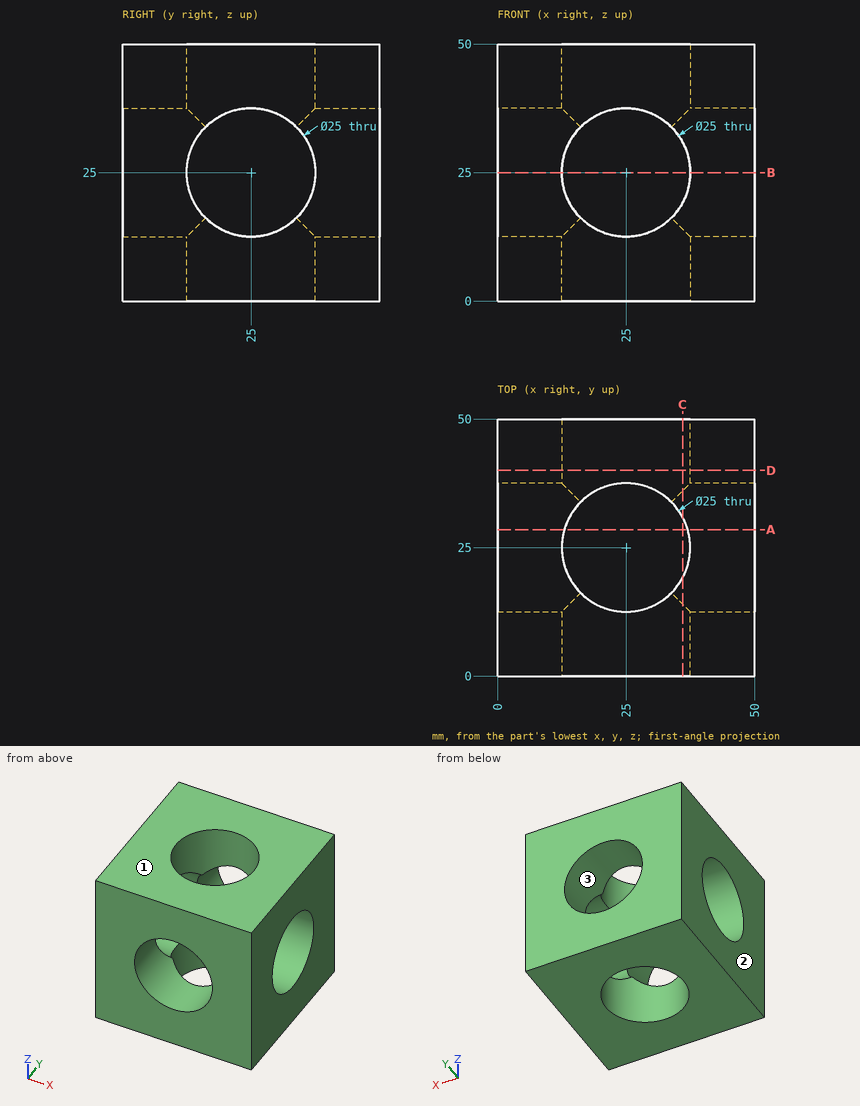
Can you work these out from the drawing? Everything is in mm from the part's minimum corner. Round coordinates to 2 decimals unless told otherwise and drop trailing zeros. Loops run counter-clockwise (first coordinate to the right, second up) from the corner with the lowest first, then second, coordinate; pieces in that order, holes last. Notation, with made-up numbers: (10, 18.25) -> (65, 18.25) arc R7 ccw to (65, 24.25) -> close; hole circle Ø11 at (78, 24). An arc over 180 degrees is marked (long way). Put each result on its own line as item: value.
Q1. I want a section at A-A on y = 28.5. Write out the boundary of the cut face in (x, z), and give its area (3 significant figures).
Checks:
outline: (0, 0) -> (13, 0) -> (13, 13) -> (0, 13) -> close; (0, 37) -> (13, 37) -> (13, 50) -> (0, 50) -> close; (37, 0) -> (50, 0) -> (50, 13) -> (37, 13) -> close; (37, 37) -> (50, 37) -> (50, 50) -> (37, 50) -> close
area: 676 mm2
Q2. I want a section at B-B on z = 25. Write out the boundary of the cut face in (x, y).
Checks:
outline: (0, 0) -> (12.5, 0) -> (12.5, 12.5) -> (0, 12.5) -> close; (0, 37.5) -> (12.5, 37.5) -> (12.5, 50) -> (0, 50) -> close; (37.5, 0) -> (50, 0) -> (50, 12.5) -> (37.5, 12.5) -> close; (37.5, 37.5) -> (50, 37.5) -> (50, 50) -> (37.5, 50) -> close
Q3. I want a section at D-D on y = 40. Write out the boundary of the cut face in (x, z), and give its area (3 significant figures).
Checks:
outline: (0, 0) -> (50, 0) -> (50, 50) -> (0, 50) -> close; hole circle Ø25 at (25, 25)
area: 2,010 mm2
Q4. Thinking about a two-plate mould opening in Z: for the marked faces 1, 2 and 3, which applies, pulls with the +Z half, pulls with the -Z half, needs draft (parallel to the pull), parting line crosses it, or undercut?
Checks:
face 1: pulls with the +Z half
face 2: needs draft
face 3: undercut
Q5. I want a section at C-C on x = 36. Write out the boundary of the cut face in (y, z).
Checks:
outline: (0, 0) -> (19.06, 0) -> (19.06, 14) arc R12.5 cw to (14, 19.06) -> (0, 19.06) -> close; (0, 30.94) -> (14, 30.94) arc R12.5 cw to (19.06, 36) -> (19.06, 50) -> (0, 50) -> close; (30.94, 0) -> (50, 0) -> (50, 19.06) -> (36, 19.06) arc R12.5 cw to (30.94, 14) -> close; (30.94, 36) arc R12.5 cw to (36, 30.94) -> (50, 30.94) -> (50, 50) -> (30.94, 50) -> close
Q6. Please list where this line runs through material, in increasing order: line 1 (Y direction, x = 25, z = 39). Write a range as from..to.
Checks:
line 1: 0..12.5, 37.5..50
